Study the drawing (mm; zero at the part's minimum x, y, z) and answer. A direction names the side the tool comes from. Round coordinates to 2 decimals unless told otherwise and drop trailing zeros. Write each loop counter-clockwise with the first axis right and the second up, starting at its lowest first coordinate (ties: lowest second). Pieces come first, ordered by that corner, then holes.
(1) A cutting plane is placed at A-A, the plane y = 4. Give the vertices of the cut face in (x, z), and give its area (3 significant figures).
(2) The mould has two halves that part along Y. Classify the marked faces 1, 2 and 3: +Y half, -Y half, draft (parallel to the pull), parting line (faces both ways), or undercut.
(3) Find the intervals of material crossed by probe 1 along X at (y, z) = (2.55, 30); probe 2 along X at (y, z) = (16, 3.05); probe 3 along Y at (x, z) = (5, 1.9), in increasing order.
(4) A cutting plane is placed at C-C, the plane x = 36. Give the vertices of the cut face in (y, z).
(5) A cutting plane is placed at D-D, the plane z = 16. Give the vertices of the cut face in (x, y), and give its area (3 significant figures).
(6) For the marked faces 4, 5, 6 and 7, determine the directions among +Z, -Z, +X, -X, +Y, -Y from which every point of the face is accessible in a straight line to the end or side of a thin tool.
(7) A cutting plane is placed at B-B, the plane z = 3. Give the vertices of the cut face in (x, y), and give its area (3 significant figures).
(8) Each of these flat-tipped pins is pushed along its axis until it touches: pin 1 Ø10 at (x, y) = (26.5, 10.5) entering from +Z; pin 2 Ø8 at (x, z) = (26, 30) entering from +Y; pin 3 Ø2.5 at (y, z) = (6, 2) entering from +X; pin 4 Ø6.5 at (x, y) = (15, 10) entering from -Z. Where does it stop, or does it pass through?
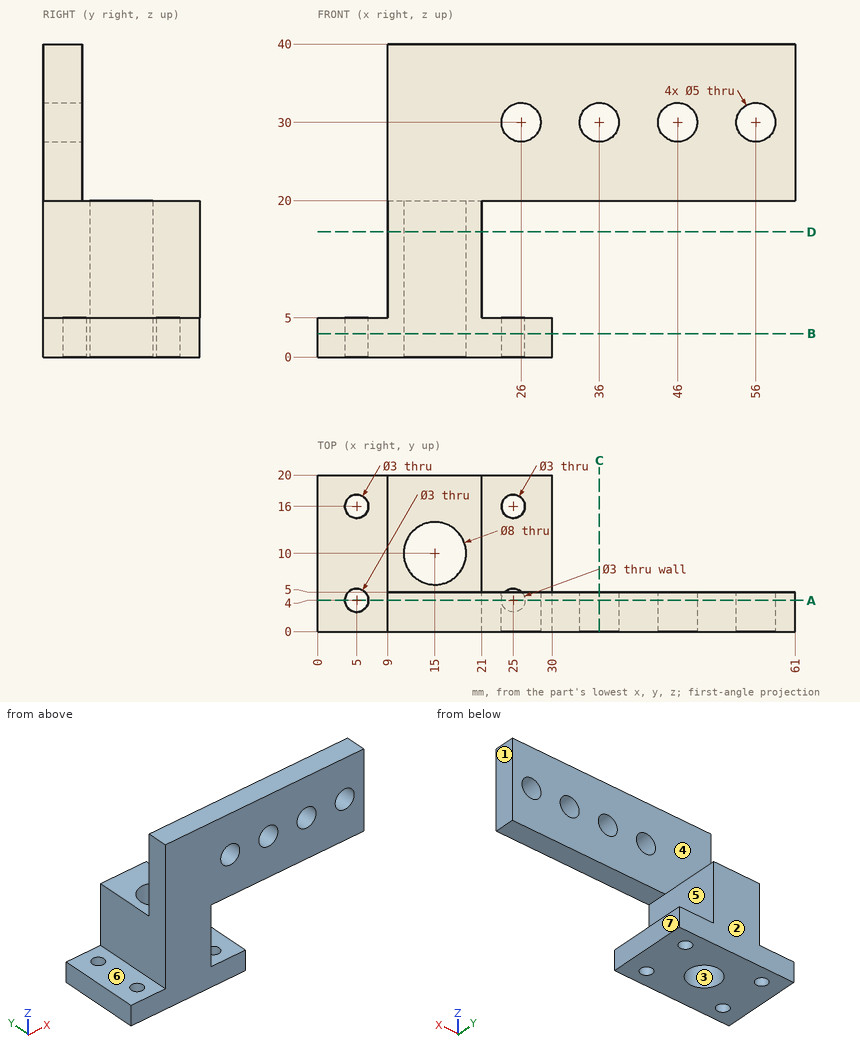
Solutions:
1. outline: (0, 0) - (3.5, 0) - (3.5, 5) - (0, 5) - close; (6.5, 0) - (23.5, 0) - (23.5, 5) - (21, 5) - (21, 20) - (61, 20) - (61, 40) - (9, 40) - (9, 5) - (6.5, 5) - close; (26.5, 0) - (30, 0) - (30, 5) - (26.5, 5) - close; hole circle Ø5 at (26, 30); hole circle Ø5 at (36, 30); hole circle Ø5 at (46, 30); hole circle Ø5 at (56, 30)
1. area: 1,260 mm2
2. face 1: draft
2. face 2: +Y half
2. face 3: undercut
3. probe 1: x = 9 to 23.5, 28.5 to 33.5, 38.5 to 43.5, 48.5 to 53.5, 58.5 to 61
3. probe 2: x = 0 to 3.5, 6.5 to 23.5, 26.5 to 30
3. probe 3: y = 0 to 2.5, 5.5 to 14.5, 17.5 to 20
4. outline: (0, 20) - (5, 20) - (5, 27.5) - (0, 27.5) - close; (0, 32.5) - (5, 32.5) - (5, 40) - (0, 40) - close
5. outline: (9, 0) - (21, 0) - (21, 20) - (9, 20) - close; hole circle Ø8 at (15, 10)
5. area: 190 mm2
6. face 4: +Z, +X, -X, +Y
6. face 5: +X, +Y, -Y
6. face 6: +Z, -X, +Y, -Y
6. face 7: -Z, +X, +Y, -Y
7. outline: (0, 0) - (30, 0) - (30, 20) - (0, 20) - close; hole circle Ø3 at (5, 4); hole circle Ø3 at (5, 16); hole circle Ø8 at (15, 10); hole circle Ø3 at (25, 4); hole circle Ø3 at (25, 16)
7. area: 521 mm2
8. pin 1: stops at z = 5
8. pin 2: stops at y = 5
8. pin 3: stops at x = 30
8. pin 4: passes through
